from build123d import *

# Parameters (mm, degrees)
F0_W     = 1
F0_H     = 10
F2_R     = 0.75
F3_DEPTH = 250
F4_DEPTH = 25


with BuildPart() as f1:
    # F0 (on Front) → F1 (revolve)
    with BuildSketch(Plane.XZ):
        with Locations((-0.5, 5)):
            Rectangle(F0_W, F0_H)
    revolve(axis=Axis((-1, 0, 5), (0, 0, 1)))

    # F2 (on Front) → F3 (cut)
    with BuildSketch(Plane.XZ):
        with Locations((-1, 7.363699)):
            Circle(F2_R)
    extrude(amount=-F3_DEPTH, mode=Mode.SUBTRACT)

    # F2 (on Front) → F4 (cut)
    with BuildSketch(Plane.XZ):
        with Locations((-1, 7.363699)):
            Circle(F2_R)
    extrude(amount=F4_DEPTH, mode=Mode.SUBTRACT)


solid = f1.part
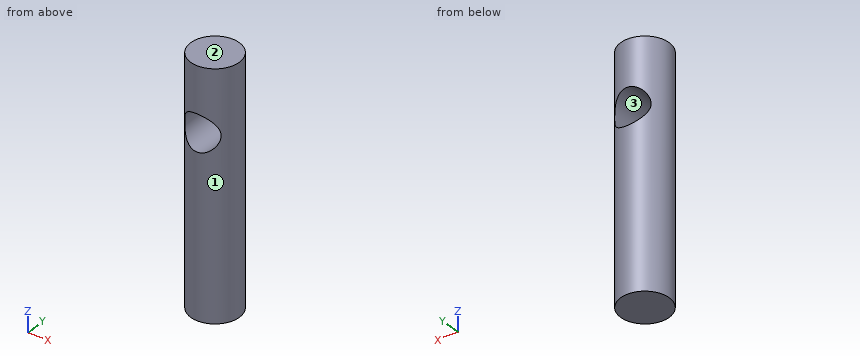
For this review, take the finished solid that the model builds, in its own axes (mm). Face numbers are marked on the shaded views. Round coordinates to 2 decimals unless told otherwise and drop trailing zeros. Order: outer loops, then holes, each group sorted by start corner. A loop starts at its lowest first (then second) coordinate and runs counter-clockwise, first axis right, second up. Notation, with made-up numbers: M -1,71.5 L 32,71.5 A7 ccw 32,82.5 Z; hole C 25.5,15.25 d8. An arc over 180 degrees is marked long. Use a Markdown table: item, result. Add a question column.
Item 1: Insertion check: pin 1 (1 mm diameter, centred on y = -1, z = 2.5, fed in from -X). The pin has a flat end and moves straight along its axis. Give the tip position at first contact, or say it passes through.
Item 2: Add section A-A, the plane x = -1. Give the boundary of the cut face in (y, z), then the cut area to 3 significant figures.
Item 3: Add section D-D, the plane z = 6.25. Give the boundary of the cut face in (x, y).
Item 4: To check wall thickness, follow line 1 along Z through (x, y) = (-1, 0.45); line 2 along X through (y, z) = (-0.05, 6); line 3 along Z through (x, y) = (-0.75, -0.6). State the ranges of each line that lie inside material, in increasing order.
Item 5: Mouldability with a two-part tool opening along Z and no side actions: class the marked faces 1, 2 and 3 as released by +Z, released by -Z, zero draft, split by the parting line, or undercut.
Item 6: Add section C-C, the plane y = -0.3. Give the boundary of the cut face in (x, z).
Item 7: Add section B-B, the plane y = -0.8. Give the boundary of the cut face in (x, z), then the cut area to 3 significant figures.
Geometry results:
| question | item | result |
|---|---|---|
| 1 | pin 1 | stops at x = -1.87 |
| 2 | outline | M -1,0 L 1,0 L 1,6.61 L -1,6.61 Z; M -1,8.11 L 1,8.11 L 1,10 L -1,10 Z |
| 2 | area | 17.0 mm² |
| 3 | outline | C -1,0 d2 |
| 4 | line 1 | z = 0 to 6.61, 8.11 to 10 |
| 4 | line 2 | x = -2 to 0 |
| 4 | line 3 | z = 0 to 6.66, 8.07 to 10 |
| 5 | face 1 | zero draft |
| 5 | face 2 | released by +Z |
| 5 | face 3 | undercut |
| 6 | outline | M -1.95,0 L -0.05,0 L -0.05,10 L -1.95,10 Z; hole C -1,7.36 d1.5 |
| 7 | outline | M -1.6,0 L -0.4,0 L -0.4,6.91 A0.75 cw -1.6,6.91 Z; M -1.6,7.81 A0.75 cw -0.4,7.81 L -0.4,10 L -1.6,10 Z |
| 7 | area | 10.4 mm² |
